Check sheet for the modelled part. Datum: model origin and axes. Units: mm. Face numbers are marked on the shaded views. Round coordinates to 2 decimals unless told otherwise and drop trailing zeros. Loops run counter-clockwise (first coordinate to the right, second up) from the corner with the lowest first, then second, coordinate; pieces in that order, holes last. Notation, with made-up numbers: (17.5, -33) - (51.5, -33) arc R13 ccw to (51.5, -12) - close; hole circle Ø10 at (40.25, 47.25). An arc over 180 degrees is marked (long way). Answer in a Markdown table with one row per item. Add a question column.
(1) Cross-section at A-A on z = 0. Enter the section's corners in (x, y), then the cut area to 3 significant figures.
(2) Cross-section at B-B on x = 0. Count the separate pieces of the cut face and the enclosed holes in it, then the cut area to 3 significant figures.
(3) Cross-section at D-D on y = 12. Enter the section's corners in (x, z).
(4) Mould release check, pull along Z, two halves, no side actions. Record for the marked faces 1 and 2: +Z half, -Z half, draft (parallel to the pull), parting line (faces both ways), or undercut.
(5) Gauge pin test, flat ends, axial feed: pin 1 (1 mm diameter, centred on x = -5.5, y = 55.5, fed in from -Z); pin 2 (3 mm diameter, centred on x = 0, y = 45, fed in from +Z); pin 3 (4 mm diameter, centred on x = 5.5, y = 15.5, fed in from -Z); pin 4 (2 mm diameter, centred on x = -2, y = 35, fed in from -Z). Record the tip position at first contact, or that the pin passes through.
(6) Thickness scan on line 1 along Y through (x, z) = (0, 6.6); line 2 along Z through (x, y) = (0, 50); line 3 along X through (y, z) = (25, -1.5). Record the ranges inside material, lowest first.
(7) Cross-section at C-C on x = 3.75. Enter the section's corners in (y, z), then the cut area to 3 significant figures.
from build123d import *

# Parameters (mm, degrees)
SKETCH_1_R               = 7
SKETCH_1_R_2             = 6
EXTRUDE_1_DEPTH          = 100
CUT_EXTRUDE_1_DEPTH      = 101.488805347
CUT_EXTRUDE_1_DEPTH_BACK = 101.488805347
SKETCH_2_R               = 1.6


with BuildPart() as part:
    # 草图1 → 凸台-拉伸1 (new body)
    with BuildSketch(Plane(origin=(0, 0, 0), x_dir=(1, 0, 0), z_dir=(0, 1, 0))):
        with Locations(Location((0, 0, 0), (0, 0, 270))):
            Circle(SKETCH_1_R)
        with Locations(Location((0, 0, 0), (0, 0, 270))):
            Circle(SKETCH_1_R_2, mode=Mode.SUBTRACT)
    extrude(amount=EXTRUDE_1_DEPTH)

    # 草图2 → 切除-拉伸1 (cut, two sides: drawn at the far end of the back side and taken through both)
    with BuildSketch(Plane.XY.offset(-CUT_EXTRUDE_1_DEPTH_BACK)):
        with Locations((0, 15)):
            Circle(SKETCH_2_R)
        with Locations((0, 30)):
            Circle(SKETCH_2_R)
        with Locations((0, 45)):
            Circle(SKETCH_2_R)
    extrude(amount=CUT_EXTRUDE_1_DEPTH + CUT_EXTRUDE_1_DEPTH_BACK, mode=Mode.SUBTRACT)


solid = part.part
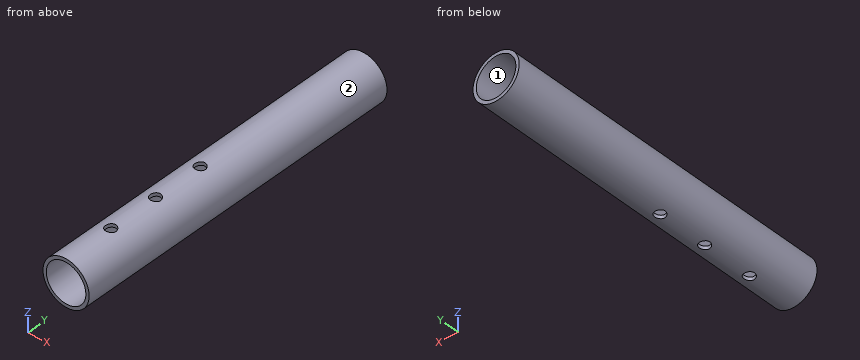
Answers:
| question | item | result |
|---|---|---|
| 1 | outline | (-7, 0) - (-6, 0) - (-6, 100) - (-7, 100) - close; (6, 0) - (7, 0) - (7, 100) - (6, 100) - close |
| 1 | area | 200 mm^2 |
| 2 | separate pieces | 8 |
| 2 | enclosed holes | 0 |
| 2 | area | 181 mm^2 |
| 3 | outline | circle Ø14 at (0, 0); hole circle Ø12 at (0, 0) |
| 4 | face 1 | undercut |
| 4 | face 2 | parting line |
| 5 | pin 1 | stops at z = -4.9 |
| 5 | pin 2 | passes through |
| 5 | pin 3 | stops at z = -6.06 |
| 5 | pin 4 | stops at z = -6.93 |
| 6 | line 1 | y = 0 to 13.4, 16.6 to 28.4, 31.6 to 43.4, 46.6 to 100 |
| 6 | line 2 | z = -7 to -6, 6 to 7 |
| 6 | line 3 | x = -6.84 to -5.81, 5.81 to 6.84 |
| 7 | outline | (0, -5.91) - (100, -5.91) - (100, -4.68) - (0, -4.68) - close; (0, 4.68) - (100, 4.68) - (100, 5.91) - (0, 5.91) - close |
| 7 | area | 245 mm^2 |
